Job drawing, mm, ordinate dimensions from the low corner. One solid piece. Coordinates: 2 decimals unless noted, no trailing zeros. Write each loop counter-clockwise with the first axis right and the second up, starting at its lowest first coordinate (ties: lowest second). Pieces come first, ordered by that corner, then holes.
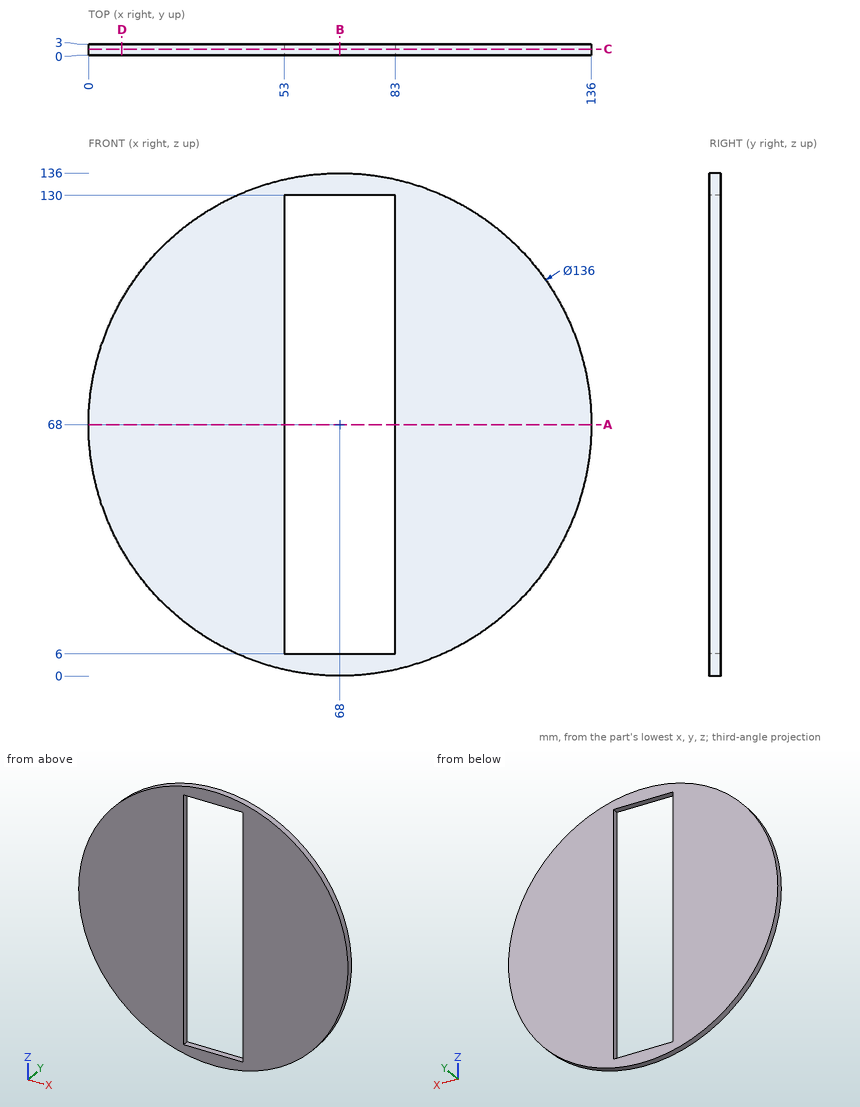
1. Saw through at B-B on x = 68. List the corners of the cut face in (y, z), plus the area to 3 significant figures.
Computed values:
outline: (0, 0) - (3, 0) - (3, 6) - (0, 6) - close; (0, 130) - (3, 130) - (3, 136) - (0, 136) - close
area: 36.0 mm2
2. Saw through at C-C on y = 1.6. List the corners of the cut face in (x, z), plus the area to 3 significant figures.
Computed values:
outline: circle Ø136 at (68, 68); hole (53, 6) - (83, 6) - (83, 130) - (53, 130) - close
area: 10,800 mm2
3. Flat gauge pins, fed straight in: pin 1 (1 mm diameter, centred on y = 2, z = 28.5, fed in from +X); pin 2 (1.5 mm diameter, centred on x = 71, y = 2, fed in from -Z); pin 3 (1.5 mm diameter, centred on y = 1, z = 75.5, fed in from +X). Where does each tip first touch, or does it go through?
Computed values:
pin 1: stops at x = 123.7
pin 2: stops at z = 0.04
pin 3: stops at x = 135.66
4. Probe line 1 along X through (y, z) = (2.5, 23.5); line 2 along Z through (x, y) = (64.5, 2.5); line 3 along X through (y, z) = (0.9, 20.5). List the from-to ranges inside material, lowest first.
Computed values:
line 1: x = 16.58 to 53, 83 to 119.42
line 2: z = 0.09 to 6, 130 to 135.91
line 3: x = 19.34 to 53, 83 to 116.66
5. Saw through at A-A on z = 68. List the corners of the cut face in (x, y).
Computed values:
outline: (0, 0) - (53, 0) - (53, 3) - (0, 3) - close; (83, 0) - (136, 0) - (136, 3) - (83, 3) - close
6. Saw through at D-D on x = 9. List the corners of the cut face in (y, z).
Computed values:
outline: (0, 34.19) - (3, 34.19) - (3, 101.81) - (0, 101.81) - close
